Geometry: final body of the model. Coordinates: model frame, mm. Face numbers are marked on the shaded views. Coordinates: 2 decimals unless noted, no trailing zeros. Write each loop counter-clockwise with the first axis right and the second up, starting at its lowest first coordinate (ties: lowest second). Pieces come first, ordered by that corner, then holes. Notation, with made-up numbers: (44, 62) - (87, 62) arc R30 ccw to (87, 101) - close; hole circle Ø3 at (48, -4). An arc over 180 degrees is marked (long way). Answer as a JSON object with one key per item and string values. Group by question number.
Item 1: Mould query, pull axis Z, two halves, no side actions, for the marked faces 1 and 2. Classes: pulls with the +Z half, pulls with the -Z half, needs draft (parallel to the pull), parting line crosses it, or undercut.
Item 2: First-contact query: pin 1 Ø0.9 at (y, z) = (-4, 2) entering from +X; pin 2 Ø1 at (y, z) = (-2, 2.5) entering from -X; pin 3 Ø1.5 at (y, z) = (6.5, 0.5) entering from +X. Flat tips, straight axial feed; report the tip coordinate or a pass-through.
Item 3: Section A-A on z = 0.5. Return loops of the section in (x, y).
Item 4: Section B-B on y = 3. Return loops of the section in (x, z).
Item 5: Line query: line 1 along Y through (x, z) = (55, 2.85); line 2 along X through (y, z) = (-3.5, 0.45); line 3 along Y through (x, z) = (120.5, 2.45) (3 decimals). Output: solid intervals per line, ascending. Write a range as from..to.
Item 6: Section C-C on x = 44.5. Return loops of the section in (y, z), and give its area (3 significant figures).
Autodesk Inventor part; units mm, degrees
ref_plane "YZ Plane" through (0, 0, 0) normal (1, 0, 0) x (0, 1, 0)
ref_plane "XZ Plane" through (0, 0, 0) normal (0, 1, 0) x (-1, 0, 0)
ref_plane "XY Plane" through (0, 0, 0) normal (0, 0, 1) x (1, 0, 0)
sketch "Sketch1" plane through (0, 0, 0) normal (0, 0, 1) x (1, 0, 0)
  line L0 (60, -6) -> (60, 0)
  line L1 (100.6, 0) -> (115.6, 0)
  line L2 (0, 0) -> (60, 0)
  line L3 (100.6, 0) -> (130.6, 0)
  line L4 (60, -6) -> (100.6, -6)
  line L5 (100.6, -6) -> (100.6, 0)
  line L6 (0, 0) -> (40, 15)
  line L7 (40, 15) -> (110.6, 15)
  line L8 (110.6, 15) -> (130.6, 0)
  dimension "d24" = 6
  dimension "d26" = 60
  dimension "d27" = 40.6
  dimension "d28" = 30
  dimension "d29" = 15
  dimension "d30" = 40
  dimension "d31" = 20
extrude "Extrusion1" add sketch "Sketch1" along normal blind 3
properties part number "Moving Ramp Inside Rail"
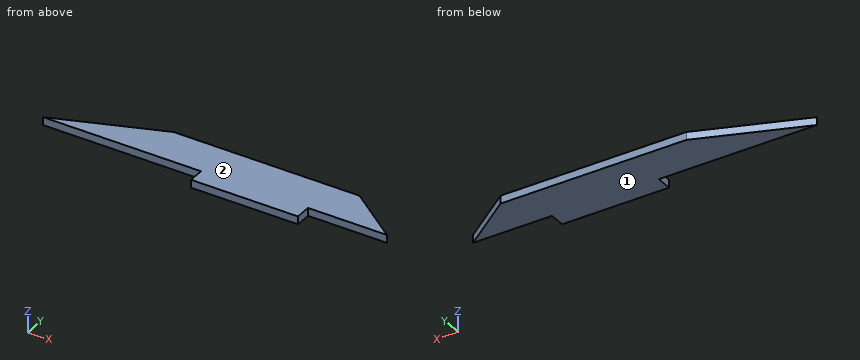
Checks:
{
 "1": {"face 1": "pulls with the -Z half", "face 2": "pulls with the +Z half"},
 "2": {"pin 1": "x = 100.6", "pin 2": "x = 60", "pin 3": "x = 122.93"},
 "3": {"outline": "(0, 0) - (60, 0) - (60, -6) - (100.6, -6) - (100.6, 0) - (130.6, 0) - (110.6, 15) - (40, 15) - close"},
 "4": {"outline": "(8, 0) - (126.6, 0) - (126.6, 3) - (8, 3) - close"},
 "5": {"line 1": "0..15", "line 2": "60..100.6", "line 3": "0..7.575"},
 "6": {"outline": "(0, 0) - (15, 0) - (15, 3) - (0, 3) - close", "area": "45.0 mm^2"}
}
